Geometry check sheet. Reference: drawing and pictorial views, mm from the part's lowest x, y, z. A direction names the side the tool comes from. Round coordinates to 2 decimals unless told otherwise and drop trailing zeros. Write each loop counter-clockwise with the first axis right and the second up, starting at its lowest first coordinate (ties: lowest second). Pieces come first, ordered by that corner, then holes. Notation, with made-up numbers: (32, 81.5) -> (78, 81.5) arc R24 cw to (78, 94.5) -> close; hole circle Ø1 at (68.25, 25). An arc over 180 degrees is marked (long way). Answer as a JSON object with one key per item and string values. Group by question number.
(1) Sectioned sample at D-D on x = 38.3. Record the cut outline in (y, z).
(2) Sectioned sample at A-A on z = 5. Record the cut outline in (x, y), and give its area (3 significant figures).
(3) Gauge pin test, flat ends, axial feed: pin 1 Ø2 at (x, z) = (50, 10) entering from +Y; pin 2 Ø3.5 at (x, z) = (51.3, 15) entering from -Y; pin 3 Ø2 at (y, z) = (18.5, 4.5) entering from -X. Record the tip position at first contact, or that the pin passes through.
(4) Scan lines: L1, parallel to X at y = 16.1, z = 5; L2, parallel to Y at x = 19, z = 15.5; L3, parallel to X at y = 24, z = 3.5. Record each from-to range of solid material in increasing order. Write a range as from..to.
(5) Sectioned sample at B-B on x = 51.3. Record the cut outline in (y, z).
(6) Set-up check for the marked faces 1, 2, 3 and 4: record each of +Z, -Z, +X, -X, +Y, -Y from which the full face is reachable in a straight line by a thin tool's end or side.
(7) Sectioned sample at C-C on z = 10. Record the cut outline in (x, y), and give its area (3 significant figures).
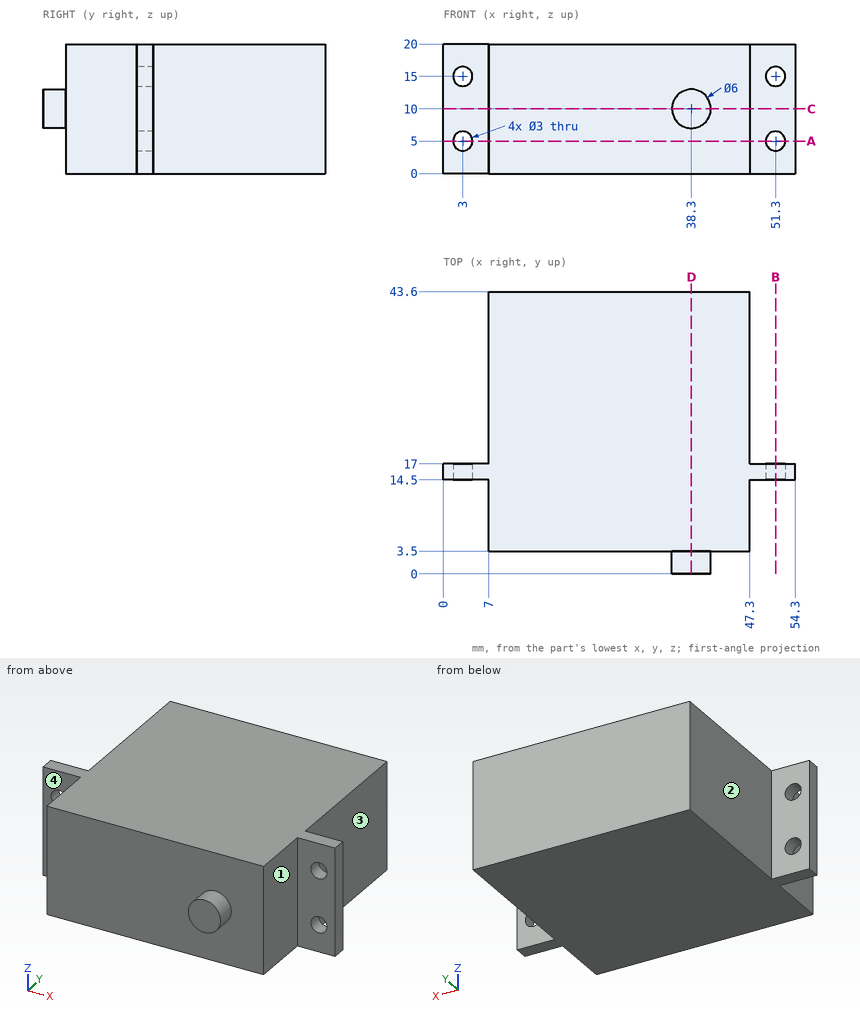
Computed values:
{
 "1": {"outline": "(0, 7) -> (3.5, 7) -> (3.5, 0) -> (43.6, 0) -> (43.6, 20) -> (3.5, 20) -> (3.5, 13) -> (0, 13) -> close"},
 "2": {"outline": "(0, 14.5) -> (1.5, 14.5) -> (1.5, 17) -> (0, 17) -> close; (4.5, 14.5) -> (7, 14.5) -> (7, 3.5) -> (47.3, 3.5) -> (47.3, 14.5) -> (49.8, 14.5) -> (49.8, 17) -> (47.3, 17) -> (47.3, 43.6) -> (7, 43.6) -> (7, 17) -> (4.5, 17) -> close; (52.8, 14.5) -> (54.3, 14.5) -> (54.3, 17) -> (52.8, 17) -> close", "area": "1,640 mm2"},
 "3": {"pin 1": "y = 17", "pin 2": "y = 14.5", "pin 3": "x = 7"},
 "4": {"L1": "0..1.5, 4.5..49.8, 52.8..54.3", "L2": "3.5..43.6", "L3": "7..47.3"},
 "5": {"outline": "(14.5, 0) -> (17, 0) -> (17, 3.5) -> (14.5, 3.5) -> close; (14.5, 6.5) -> (17, 6.5) -> (17, 13.5) -> (14.5, 13.5) -> close; (14.5, 16.5) -> (17, 16.5) -> (17, 20) -> (14.5, 20) -> close"},
 "6": {"face 1": "+Z, -Z, +X, -Y", "face 2": "+Z, -Z, -X, +Y", "face 3": "+Z, -Z, +X, +Y", "face 4": "+Z, -Z, -X, -Y"},
 "7": {"outline": "(0, 14.5) -> (7, 14.5) -> (7, 3.5) -> (35.3, 3.5) -> (35.3, 0) -> (41.3, 0) -> (41.3, 3.5) -> (47.3, 3.5) -> (47.3, 14.5) -> (54.3, 14.5) -> (54.3, 17) -> (47.3, 17) -> (47.3, 43.6) -> (7, 43.6) -> (7, 17) -> (0, 17) -> close", "area": "1,670 mm2"}
}
